```python
from build123d import *

# Parameters (mm, degrees)
ESQUISSE1_W             = 30
ESQUISSE1_H             = 30
BOSS_EXTRU_1_DEPTH      = 15
CHANFREIN1_START        = 19.052558883
CHANFREIN1_OUTLINE_W    = 17
CHANFREIN1_OUTLINE_H    = 20
CHANFREIN1_DEPTH        = 7.947441117
CHANFREIN2_START        = 19.052558883
CHANFREIN2_OUTLINE_W    = 17
CHANFREIN2_OUTLINE_H    = 20
CHANFREIN2_DEPTH        = 7.947441117
ESQUISSE2_R             = 3.25
ENL_V_MAT_EXTRU_1_DEPTH = 10
CHANFREIN4_START        = -27
CHANFREIN4_OUTLINE_W    = 17
CHANFREIN4_OUTLINE_H    = 20
CHANFREIN4_DEPTH        = 7.947441117
CHANFREIN5_START        = -27
CHANFREIN5_OUTLINE_W    = 17
CHANFREIN5_OUTLINE_H    = 20
CHANFREIN5_DEPTH        = 7.947441117
CHANFREIN3_SIZE         = 8
ESQUISSE3_R             = 3.25
ENL_V_MAT_EXTRU_2_DEPTH = 10
ESQUISSE4_R             = 104
ENL_V_MAT_EXTRU_3_DEPTH = 20
ESQUISSE5_R             = 1.6
ENL_V_MAT_EXTRU_4_DEPTH = 20
ENL_V_MAT_EXTRU_5_DEPTH = 2


with BuildPart() as part:
    # Esquisse1 → Boss.-Extru.1 (new, symmetric)
    with BuildSketch(Plane.XY):
        Rectangle(ESQUISSE1_W, ESQUISSE1_H)
    extrude(amount=BOSS_EXTRU_1_DEPTH, both=True)

    # Chanfrein1: read off the stored shape, not the designer's step
    # Chanfrein1 outline → Chanfrein1 (cut)
    with BuildSketch(Plane(origin=(0, 0, 0), x_dir=(0.8164965809277258, 0.40824829046386313, 0.40824829046386313), z_dir=(0.5773502691896258, -0.5773502691896258, -0.5773502691896258)).offset(CHANFREIN1_START)):
        with Locations((-2.5, 0)):
            Rectangle(CHANFREIN1_OUTLINE_W, CHANFREIN1_OUTLINE_H)
    extrude(amount=CHANFREIN1_DEPTH, mode=Mode.SUBTRACT)

    # Chanfrein2: read off the stored shape, not the designer's step
    # Chanfrein2 outline → Chanfrein2 (cut)
    with BuildSketch(Plane(origin=(0, 0, 0), x_dir=(0.8164965809277258, 0.40824829046386313, -0.40824829046386313), z_dir=(0.5773502691896258, -0.5773502691896258, 0.5773502691896258)).offset(CHANFREIN2_START)):
        with Locations((-2.5, 0)):
            Rectangle(CHANFREIN2_OUTLINE_W, CHANFREIN2_OUTLINE_H)
    extrude(amount=CHANFREIN2_DEPTH, mode=Mode.SUBTRACT)

    # Esquisse2 → Enlèv. mat.-Extru.1 (cut)
    with BuildSketch(Plane(origin=(11, -11, -11), x_dir=(-0.40824829046386296, 0.4082482904638631, -0.816496580927726), z_dir=(0.5773502691896257, -0.5773502691896258, -0.5773502691896258))):
        with Locations(Location((0, 0, 0), (0, 0, 30))):
            Circle(ESQUISSE2_R)
    enl_v_mat_extru_1 = extrude(amount=-ENL_V_MAT_EXTRU_1_DEPTH, mode=Mode.SUBTRACT)

    # Symétrie3: Enlèv. mat.-Extru.1 across plane
    add(enl_v_mat_extru_1.mirror(Plane.XY), mode=Mode.SUBTRACT)

    # Chanfrein4: read off the stored shape, not the designer's step
    # Chanfrein4 outline → Chanfrein4 (cut)
    with BuildSketch(Plane(origin=(0, 0, 0), x_dir=(0.8164965809277258, -0.40824829046386313, 0.40824829046386313), z_dir=(0.5773502691896258, 0.5773502691896258, -0.5773502691896258)).offset(CHANFREIN4_START)):
        with Locations((2.5, 0)):
            Rectangle(CHANFREIN4_OUTLINE_W, CHANFREIN4_OUTLINE_H)
    extrude(amount=CHANFREIN4_DEPTH, mode=Mode.SUBTRACT)

    # Chanfrein5: read off the stored shape, not the designer's step
    # Chanfrein5 outline → Chanfrein5 (cut)
    with BuildSketch(Plane(origin=(0, 0, 0), x_dir=(0.8164965809277258, -0.40824829046386313, -0.40824829046386313), z_dir=(0.5773502691896258, 0.5773502691896258, 0.5773502691896258)).offset(CHANFREIN5_START)):
        with Locations((2.5, 0)):
            Rectangle(CHANFREIN5_OUTLINE_W, CHANFREIN5_OUTLINE_H)
    extrude(amount=CHANFREIN5_DEPTH, mode=Mode.SUBTRACT)

    # Chanfrein3
    chanfrein3_edges = [part.edges().sort_by_distance(p)[0] for p in [
        (-15, -15, 0),
    ]]
    chamfer(chanfrein3_edges, length=CHANFREIN3_SIZE)

    # Esquisse3 → Enlèv. mat.-Extru.2 (cut)
    with BuildSketch(Plane(origin=(-11, -11, 0), x_dir=(0, 0, 1), z_dir=(-0.7071067811865487, -0.7071067811865465, 0))):
        with Locations(Location((0, 0, 0), (0, 0, 270))):
            Circle(ESQUISSE3_R)
    extrude(amount=-ENL_V_MAT_EXTRU_2_DEPTH, mode=Mode.SUBTRACT)

    # Esquisse4 → Enlèv. mat.-Extru.3 (cut)
    with BuildSketch(Plane.XY.offset(15)):
        with Locations((0, 108)):
            Circle(ESQUISSE4_R)
    extrude(amount=-ENL_V_MAT_EXTRU_3_DEPTH, mode=Mode.SUBTRACT)

    # Esquisse5 → Enlèv. mat.-Extru.4 (cut)
    with BuildSketch(Plane.XY.offset(-5)):
        with Locations((-5, 9)):
            Circle(ESQUISSE5_R)
        with Locations((5, 9)):
            Circle(ESQUISSE5_R)
    extrude(amount=-ENL_V_MAT_EXTRU_4_DEPTH, mode=Mode.SUBTRACT)

    # Esquisse6 → Enlèv. mat.-Extru.5 (cut)
    with BuildSketch(Plane(origin=(0, 0, -15), x_dir=(-1, 0, 0), z_dir=(0, 0, -1))):
        Polygon((-3.383419246, 11.8), (-6.616580754, 11.8), (-8.233161507, 9), (-6.616580754, 6.2), (-3.383419246, 6.2), (-1.766838493, 9), align=None)
        Polygon((6.616580754, 11.8), (3.383419246, 11.8), (1.766838493, 9), (3.383419246, 6.2), (6.616580754, 6.2), (8.233161507, 9), align=None)
    extrude(amount=-ENL_V_MAT_EXTRU_5_DEPTH, mode=Mode.SUBTRACT)


solid = part.part
```
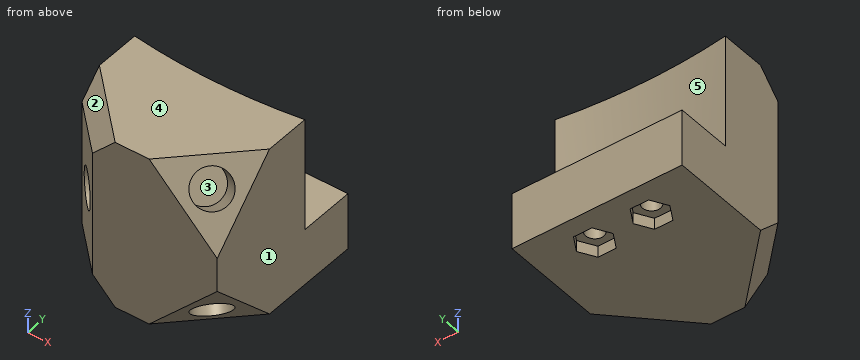
CAD build for the part. Positions are in the model's coordinates, mm. Face numbers are marked on the shaded views. A direction names the side the tool comes from. Round coordinates to 2 decimals unless told otherwise and drop trailing zeros. Loops run counter-clockwise (first coordinate to the right, second up) from the corner with the lowest first, then second, coordinate; pieces in that order, holes last. Notation, with made-up numbers: (68.25, 45) - (120.25, 45) arc R26 ccw to (120.25, 61) - close; hole circle Ø11 at (43, 11.25). An arc over 180 degrees is marked (long way). Return JSON: item names as keys, results as strings. Group by question number.
Q1. Flat gauge pins, fed straight in: pin 1 Ø3.5 at (x, y) = (5, 9) entering from +Z; pin 2 Ø3 at (x, y) = (-5.5, 8) entering from -Z. Where does each tip first touch, or does it go through?
Q2. Band-saw the part on A-A on y = 8.5. Give the cut face in (x, z).
Q3. Tool access for the marked faces 4 and 5: list every direction of +Z, -Z, +X, -X, +Y, -Y with a clear straight run to the whole face (end or side of a thin tool).
Q4. Two-plate mould, pull along X, no slides. Class the marked faces 1, 2 and 3: +X half, -X half, draft (parallel to the pull), parting line (faces both ways), or undercut.
Q5. Drill centre lines: line 1 along Z through (x, y) = (9, -6.5); line 2 along Y through (x, z) = (-5, -7.25); line 3 along Y through (x, z) = (5, -9). Where is each one in solid material? Low to high. Write a range as [from, to].
Q6. Band-saw the part on C-C on z = 1.5. Give the cut face in (x, y), plus the area to 3 significant figures.
Q7. Band-saw the part on B-B on x = -5. Give the number of separate pieces and of enclosed holes in the cut face, plus the area to 3 significant figures.
Solutions:
{
 "1": {"pin 1": "stops at z = -5", "pin 2": "stops at z = -13"},
 "2": {"outline": "(-15, -15) - (-7.94, -15) - (-7.94, -13) - (-6.52, -13) - (-6.52, -5) - (-15, -5) - close; (-3.48, -13) - (-2.06, -13) - (-2.06, -15) - (2.06, -15) - (2.06, -13) - (3.48, -13) - (3.48, -5) - (-3.48, -5) - close; (6.52, -13) - (7.94, -13) - (7.94, -15) - (15, -15) - (15, -5) - (6.52, -5) - close"},
 "3": {"face 4": "+Z, +X, -X, +Y, -Y", "face 5": "+Z, +Y"},
 "4": {"face 1": "+X half", "face 2": "-X half", "face 3": "undercut"},
 "5": {"line 1": "z = [-15, -11.09], [-4.41, 4.41], [11.09, 15]", "line 2": "y = [-15, 7.4], [10.6, 15]", "line 3": "y = [-15, -8.96], [-5.04, 7.4], [10.6, 15]"},
 "6": {"outline": "(-15, -7) - (-13.04, -8.96) - (-5.97, -1.89) - (-1.89, -5.97) - (-8.96, -13.04) - (-7, -15) - (15, -15) - (15, 5.09) arc R104 cw to (-15, 5.09) - close", "area": "491 mm^2"},
 "7": {"separate pieces": "2", "enclosed holes": "1", "area": "605 mm^2"}
}
